CAD build for the part. Positions are in the model's coordinates, mm. A direction names the side the tool comes from. Round coordinates to 2 decimals unless told otherwise and drop trailing zeros. Order: outer loops, then holes, each group sorted by start corner. A loop starts at its lowest first (then second) coordinate and runs counter-clockwise, first axis right, second up. Notation, with made-up numbers: M 85,86.5 L 142,86.5 A16 cw 142,106.5 Z; hole C 76.5,35.5 d3. An arc over 180 degrees is marked long. Answer as a JSON object with one key per item and string values.
```python
from build123d import *

# Parameters (mm, degrees)
F3_R      = 4.7
F4_DEPTH  = 37
F8_DEPTH  = 37
F6_R      = 4.7
F6_R_2    = 4
F9_DEPTH  = 25
F7_R      = 4.7
F7_R_2    = 4
F10_DEPTH = 18
F11_R     = 2.75
F12_DEPTH = 4.701


# Not quite as in the source:
# - ends of sketch curves that miss each other by under 0.0002 mm in the source are joined


with BuildPart() as f4:
    # F3 (on Front) → F4 (new body)
    with BuildSketch(Plane.XZ):
        Circle(F3_R)
    extrude(amount=F4_DEPTH)

    # F5 (on face) → F8 (cut, through all)
    with BuildSketch(Plane.XZ.offset(37)):
        with BuildLine():
            Line((-1.25, -3.8), (0, -3.8))
            Line((0, -3.8), (1.25, -3.8))
            Line((1.25, -3.8), (1.25, -3.7))
            ThreePointArc((1.25, -3.7), (1.3085786438, -3.5585786438), (1.45, -3.5))
            Line((1.45, -3.5), (2, -3.5))
            Line((2, -3.5), (2, -3.05))
            ThreePointArc((2, -3.05), (2.0585786438, -2.9085786438), (2.2, -2.85))
            Line((2.2, -2.85), (3.15, -2.85))
            Line((3.15, -2.85), (3.15, -2.15))
            Line((3.15, -2.15), (2.2, -2.15))
            ThreePointArc((2.2, -2.15), (2.0585786438, -2.0914213562), (2, -1.95))
            Line((2, -1.95), (2, -1.887459))
            ThreePointArc((2, -1.887459), (2.1033535752, -1.771554046), (2.2, -1.65))
            Line((2.2, -1.65), (3.75, -1.65))
            Line((3.75, -1.65), (3.75, 0))
            Line((3.75, 0), (3.75, 1.65))
            Line((3.75, 1.65), (2.2, 1.65))
            ThreePointArc((2.2, 1.65), (2.1033535752, 1.771554046), (1.9999998047, 1.8874588157))
            Line((1.9999998047, 1.8874588157), (2, 1.95))
            ThreePointArc((2, 1.95), (2.0585786438, 2.0914213562), (2.2, 2.15))
            Line((2.2, 2.15), (3.15, 2.15))
            Line((3.15, 2.15), (3.15, 2.85))
            Line((3.15, 2.85), (2.2, 2.85))
            ThreePointArc((2.2, 2.85), (2.0585786438, 2.9085786438), (2, 3.05))
            Line((2, 3.05), (2, 3.5))
            Line((2, 3.5), (1.45, 3.5))
            ThreePointArc((1.45, 3.5), (1.3085786438, 3.5585786438), (1.25, 3.7))
            Line((1.25, 3.7), (1.25, 3.8))
            Line((1.25, 3.8), (0, 3.8))
            Line((0, 3.8), (-1.25, 3.8))
            Line((-1.25, 3.8), (-1.25, 3.7))
            ThreePointArc((-1.25, 3.7), (-1.3085786438, 3.5585786438), (-1.45, 3.5))
            Line((-1.45, 3.5), (-2, 3.5))
            Line((-2, 3.5), (-2, 3.05))
            ThreePointArc((-2, 3.05), (-2.0585786438, 2.9085786438), (-2.2, 2.85))
            Line((-2.2, 2.85), (-3.15, 2.85))
            Line((-3.15, 2.85), (-3.15, 2.15))
            Line((-3.15, 2.15), (-2.2, 2.15))
            ThreePointArc((-2.2, 2.15), (-2.0585786438, 2.0914213562), (-2, 1.95))
            Line((-2, 1.95), (-2, 1.887459))
            ThreePointArc((-2, 1.887459), (-2.1033535752, 1.771554046), (-2.2, 1.65))
            Line((-2.2, 1.65), (-3.75, 1.65))
            Line((-3.75, 1.65), (-3.75, 0))
            Line((-3.75, 0), (-3.75, -1.65))
            Line((-3.75, -1.65), (-2.2, -1.65))
            ThreePointArc((-2.2, -1.65), (-2.1033535752, -1.771554046), (-1.9999998047, -1.8874588157))
            Line((-1.9999998047, -1.8874588157), (-2, -1.95))
            ThreePointArc((-2, -1.95), (-2.0585786438, -2.0914213562), (-2.2, -2.15))
            Line((-2.2, -2.15), (-3.15, -2.15))
            Line((-3.15, -2.15), (-3.15, -2.85))
            Line((-3.15, -2.85), (-2.2, -2.85))
            ThreePointArc((-2.2, -2.85), (-2.0585786438, -2.9085786438), (-2, -3.05))
            Line((-2, -3.05), (-2, -3.5))
            Line((-2, -3.5), (-1.45, -3.5))
            ThreePointArc((-1.45, -3.5), (-1.3085786438, -3.5585786438), (-1.25, -3.7))
            Line((-1.25, -3.7), (-1.25, -3.8))
        make_face()
    extrude(amount=-F8_DEPTH, mode=Mode.SUBTRACT)

    # F6 (on face) → F9 (join)
    with BuildSketch(Plane.XZ.offset(37)):
        Circle(F6_R)
        Circle(F6_R_2, mode=Mode.SUBTRACT)
    extrude(amount=F9_DEPTH)

    # F7 (on face) → F10 (join)
    with BuildSketch(Plane(origin=(0, 0, 0), x_dir=(-1, 0, 0), z_dir=(0, 1, 0))):
        Circle(F7_R)
        Circle(F7_R_2, mode=Mode.SUBTRACT)
    extrude(amount=F10_DEPTH)

    # F11 (on Right) → F12 (cut, through all)
    with BuildSketch(Plane.YZ):
        with Locations((-56, 0)):
            Circle(F11_R)
    extrude(amount=-F12_DEPTH, mode=Mode.SUBTRACT)


solid = f4.part
```
Item 1: Saw through at D-D on y = -56. List the corners of the cut face in (x, z), and give its area (3 significant figures).
Worked answers:
{"outline": "M -3.81,-2.75 A4.7 ccw long -3.81,2.75 L -2.9,2.75 A4 cw long -2.9,-2.75 Z", "area": "15.0 mm2"}
Item 2: Drop flat-ended pins along their axis: pin 1 Ø0.8 at (y, z) = (-23, -2.5) entering from -X; pin 2 Ø3 at (x, y) = (-2, 3.5) entering from +Z; pin 3 Ø2 at (x, y) = (2, -31) entering from -Z. Give the stop position or say it passes through.
Worked answers:
{"pin 1": "stops at x = -4.2", "pin 2": "stops at z = 4.67", "pin 3": "stops at z = -4.59"}
Item 3: Saw through at B-B on x = 0. List the corners of the cut face in (y, z).
Worked answers:
{"outline": "M -62,-4.7 L 18,-4.7 L 18,-4 L 0,-4 L 0,-3.8 L -37,-3.8 L -37,-4 L -62,-4 Z; M -62,4 L -37,4 L -37,3.8 L 0,3.8 L 0,4 L 18,4 L 18,4.7 L -62,4.7 Z"}
Item 4: Wall check: line 1 along X through (y, z) = (-38, -3.5); line 2 along X through (y, z) = (7, 0). Give the ranges that are in metal, low to high. Write a range as [from, to].
Worked answers:
{"line 1": "x = [-3.14, -1.94], [1.94, 3.14]", "line 2": "x = [-4.7, -4], [4, 4.7]"}
Item 5: Saw through at C-C on y = 11.5. List the corners of the cut face in (x, z), and give its area (3 significant figures).
Worked answers:
{"outline": "C 0,0 d9.4; hole C 0,0 d8", "area": "19.1 mm2"}
Item 6: Saw through at A-A on z = 0. List the corners of the cut face in (x, y), and give its area (3 significant figures).
Worked answers:
{"outline": "M -4.7,-62 L -4,-62 L -4,-58.75 L -4.7,-58.75 Z; M -4.7,-53.25 L -4,-53.25 L -4,-37 L -3.75,-37 L -3.75,0 L -4,0 L -4,18 L -4.7,18 Z; M 3.75,-37 L 4,-37 L 4,-62 L 4.7,-62 L 4.7,18 L 4,18 L 4,0 L 3.75,0 Z", "area": "127 mm2"}
Item 7: Two-plate mould, pull along Z, no slides. Class faces 4 (the flat face through (2, -62, 4)), 5 (the cylindrical face through (0.867, 8.874, -3.905)): released by +Z, released by -Z, zero draft, split by the parting line, or undercut.
Worked answers:
{"face 4": "zero draft", "face 5": "undercut"}
Item 8: 3-axis set-ups, long thin cutter, end or side, ignore diameter. For faces 1 (the cylindrical face through (3.815, -49.325, 1.201)), 2 (the flat face through (0, -19, 3.8)), 3 (the flat face through (-3.75, -19, 0)): which of +Z, -Z, +X, -X, +Y, -Y reach the whole face in a straight line?
Worked answers:
{"face 1": "-Y", "face 2": "+Y, -Y", "face 3": "none"}
